from build123d import *

# Parameters (mm, degrees)
BOSS_EXTRUDE1_DEPTH = 300
SKETCH2_R           = 2.6
CUT_EXTRUDE1_DEPTH  = 15


with BuildPart() as part:
    # Sketch1 → Boss-Extrude1 (new body)
    with BuildSketch(Plane.XY):
        Polygon((-8, 6.585786438), (-4, 2.585786438), (-4, -2.585786438), (-8, -6.585786438), (-8, -3.1), (-10, -3.1), (-10, -10), (-3.1, -10), (-3.1, -8), (-6.585786438, -8), (-2.585786438, -4), (2.585786438, -4), (6.585786438, -8), (3.1, -8), (3.1, -10), (10, -10), (10, -3.1), (8, -3.1), (8, -6.585786438), (4, -2.585786438), (4, 2.585786438), (8, 6.585786438), (8, 3.1), (10, 3.1), (10, 10), (3.1, 10), (3.1, 8), (6.585786438, 8), (2.585786438, 4), (-2.585786438, 4), (-6.585786438, 8), (-3.1, 8), (-3.1, 10), (-10, 10), (-10, 3.1), (-8, 3.1), align=None)
    extrude(amount=BOSS_EXTRUDE1_DEPTH)

    # Sketch2 → Cut-Extrude1 (cut, through all)
    with BuildSketch(Plane.ZY.offset(4)):
        with Locations((150, 0)):
            Circle(SKETCH2_R)
    extrude(amount=-CUT_EXTRUDE1_DEPTH, mode=Mode.SUBTRACT)


solid = part.part
The model under review builds one solid part; all positions refer to its coordinate system, in mm. A direction names the side the tool comes from. Give positions to 0.01 mm unless a question says otherwise; leave off trailing zeros. Order: outer loops, then holes, each group sorted by start corner. A loop starts at its lowest first (then second) coordinate and runs counter-clockwise, first axis right, second up. Notation, with made-up numbers: M 58.5,80 L 68.5,80 A16 ccw 68.5,89 Z; hole C 82,64 d10. An arc over 180 degrees is marked long. Answer in a Markdown table with one row per item. Add a question column.
1. Machinability: for faces 1 (the flat face through (0, 0, 300)), 2 (the flat face through (4, 0, 224)), 3 (the flat face through (-4, 0, 224)), 4 (the flat face through (0, 4, 148)), which of the approach directions +Z, -Z, +X, -X, +Y, -Y give a long, thin tool a straight path to every point of the face, cutting with its end or side? Answer none if there is none.
2. Add section A-A on y = 0. State the section outline as (x, z) points.
3. For pin 1 Ø2.5 at (y, z) = (-1, 243) entering from +X; pin 2 Ø4 at (x, z) = (0.5, 159.5) entering from +Y; pin 3 Ø5.5 at (y, z) = (0, 66.5) entering from +X; pin 4 Ø1.5 at (x, y) = (2, 6.5) entering from -Z, all flat-tipped, find the tip position at first contact; note any pin that passes through.
4. Mouldability with a two-part tool opening along Y and no side actions: class faces 5 (the flat face through (-7, 10, 148)), 6 (the flat face through (0, -4, 148)), 7 (the flat face through (10, 7, 148)), 8 (the flat face through (4, 0, 74)) as released by +Y, released by -Y, zero draft, split by the parting line, or undercut.
5. To check wall thickness, follow line 1 along Z through (x, y) = (-1.5, 0); line 2 along X through (y, z) = (6.25, 46); line 3 along Y through (x, z) = (9.25, 200.5). State the ranges of each line that lie inside material, in increasing order.
The answers:
| question | item | result |
|---|---|---|
| 1 | face 1 | +Z, +X, -X, +Y, -Y |
| 1 | face 2 | +Z, -Z, +X |
| 1 | face 3 | +Z, -Z, -X |
| 1 | face 4 | +Z, -Z, +Y |
| 2 | outline | M -4,0 L 4,0 L 4,147.4 L -4,147.4 Z; M -4,152.6 L 4,152.6 L 4,300 L -4,300 Z |
| 3 | pin 1 | x = 4 |
| 3 | pin 2 | y = 4 |
| 3 | pin 3 | x = 4.16 |
| 3 | pin 4 | through |
| 4 | face 5 | released by +Y |
| 4 | face 6 | released by -Y |
| 4 | face 7 | zero draft |
| 4 | face 8 | undercut |
| 5 | line 1 | 0 to 147.4, 152.6 to 300 |
| 5 | line 2 | -10 to -8, -7.66 to -4.84, 4.84 to 7.66, 8 to 10 |
| 5 | line 3 | -10 to -3.1, 3.1 to 10 |
